For this review, take the finished solid that the model builds, in its own axes (mm). A direction names the side the tool comes from. Round coordinates to 2 decimals unless told otherwise and drop trailing zeros. Write each loop counter-clockwise with the first axis right and the second up, starting at its lowest first coordinate (ties: lowest second). Pieces come first, ordered by that corner, then holes. Notation, with made-up numbers: M 50,79.5 L 108,79.5 A20 ccw 108,84.5 Z; hole C 84.25,48.5 d11. An arc over 180 degrees is marked long. Use one line per item in the form item = value. Start each with the question number.
Item 1: Add section B-B (x = -8.25). State the section outline as (y, z) points.
Item 2: Add section D-D (x = 10.25). State the section outline as (y, z) points, and give its area (3 significant figures).
Item 3: For line 1 (Y direction, x = 7, z = 2.5); line 2 (Y direction, x = 9, z = 1.6); line 3 (Y direction, x = 2.75, z = 0.4), list the stretches that pass through material, from the lowest coordinate up. Write a range as [from, to].
Item 4: Add section A-A (z = 1.55). Count the separate pieces of the cut face and the enclosed holes in it, and give its area (3 significant figures).
Item 5: Add section C-C (y = 1.5). State the section outline as (x, z) points (3 decimals).
Item 6: Draft analysis for pull direction X (two halves, no side actions). For faces 4 (the flat face through (7, 0, 3.5)), 5 (the cylindrical face through (11.859, 22.797, 1.726)), 6 (the flat face through (-0.1, 1.2, 2)), state which applies: released by +X, released by -X, zero draft, split by the parting line, or undercut.
Item 7: For faces 1 (the flat face through (0, -24, 2)), 2 (the flat face through (-4.25, 0, 3)), 3 (the flat face through (0, -5, 1)), list the 3-axis set-ups (+Z, -Z, +X, -X, +Y, -Y) from which the entire face can be reached by the end or side of a thin tool; tool diameter is ignored.
from build123d import *

# Parameters (mm, degrees)
F0_R     = 1.75
F0_W     = 12
F0_H     = 10
F1_DEPTH = 2
F2_R     = 1.75
F3_DEPTH = 1.5
F4_R     = 1.125
F5_DEPTH = 60
F6_W     = 8.5
F6_H     = 2
F7_DEPTH = 5


with BuildPart() as f1:
    # F0 (on Top) → F1 (new body)
    with BuildSketch(Plane.XY):
        with BuildLine():
            ThreePointArc((-13, -20), (-11.828427, -22.828427), (-9, -24))
            Line((-9, -24), (9, -24))
            ThreePointArc((9, -24), (11.828427, -22.828427), (13, -20))
            Line((13, -20), (13, 20))
            ThreePointArc((13, 20), (11.828427, 22.828427), (9, 24))
            Line((9, 24), (-9, 24))
            ThreePointArc((-9, 24), (-11.828427, 22.828427), (-13, 20))
            Line((-13, 20), (-13, -20))
        make_face()
        with Locations((-9, -20)):
            Circle(F0_R, mode=Mode.SUBTRACT)
        with Locations((-7, -7)):
            Circle(F0_R, mode=Mode.SUBTRACT)
        with Locations((9, -20)):
            Circle(F0_R, mode=Mode.SUBTRACT)
        with Locations((7, -7)):
            Circle(F0_R, mode=Mode.SUBTRACT)
        with Locations((-7, 7)):
            Circle(F0_R, mode=Mode.SUBTRACT)
        with Locations((-9, 20)):
            Circle(F0_R, mode=Mode.SUBTRACT)
        Rectangle(F0_W, F0_H, mode=Mode.SUBTRACT)
        with Locations((7, 7)):
            Circle(F0_R, mode=Mode.SUBTRACT)
        with Locations((9, 20)):
            Circle(F0_R, mode=Mode.SUBTRACT)
    extrude(amount=F1_DEPTH)

    # F2 (on face) → F3 (join)
    with BuildSketch(Plane.XY.offset(2)):
        with BuildLine():
            ThreePointArc((-13, -20), (-11.828427, -22.828427), (-9, -24))
            Line((-9, -24), (9, -24))
            ThreePointArc((9, -24), (11.828427, -22.828427), (13, -20))
            Line((13, -20), (13, 20))
            ThreePointArc((13, 20), (11.828427, 22.828427), (9, 24))
            Line((9, 24), (-9, 24))
            ThreePointArc((-9, 24), (-11.828427, 22.828427), (-13, 20))
            Line((-13, 20), (-13, -20))
        make_face()
        with Locations((-9, -20)):
            Circle(F2_R, mode=Mode.SUBTRACT)
        with Locations((-7, -7)):
            Circle(F2_R, mode=Mode.SUBTRACT)
        with Locations((9, -20)):
            Circle(F2_R, mode=Mode.SUBTRACT)
        with Locations((7, -7)):
            Circle(F2_R, mode=Mode.SUBTRACT)
        with Locations((-7, 7)):
            Circle(F2_R, mode=Mode.SUBTRACT)
        with Locations((-9, 20)):
            Circle(F2_R, mode=Mode.SUBTRACT)
        with Locations((7, 7)):
            Circle(F2_R, mode=Mode.SUBTRACT)
        with Locations((9, 20)):
            Circle(F2_R, mode=Mode.SUBTRACT)
    extrude(amount=F3_DEPTH)


with BuildPart() as f5:
    # F4 (on face) → F5 (new body)
    with BuildSketch(Plane.XZ.offset(24)):
        with Locations((0, 3.5)):
            Circle(F4_R)
    extrude(amount=-F5_DEPTH)


with BuildPart() as f7:
    # F6 (on face) → F7 (new body)
    with BuildSketch(Plane.XY.offset(3.5)):
        Rectangle(F6_W, F6_H)
    extrude(amount=-F7_DEPTH)


with BuildPart() as f1_1:
    add(f1.part)

    # F8: cut F5, F7
    add(f5.part, mode=Mode.SUBTRACT)
    add(f7.part, mode=Mode.SUBTRACT)


solid = f1_1.part
Calculated:
q1.outline = M -24,0 L -21.58,0 L -21.58,3.5 L -24,3.5 Z; M -18.42,0 L -8.22,0 L -8.22,3.5 L -18.42,3.5 Z; M -5.78,0 L 5.78,0 L 5.78,3.5 L -5.78,3.5 Z; M 8.22,0 L 18.42,0 L 18.42,3.5 L 8.22,3.5 Z; M 21.58,0 L 24,0 L 24,3.5 L 21.58,3.5 Z
q2.outline = M -23.8,0 L -21.22,0 L -21.22,3.5 L -23.8,3.5 Z; M -18.78,0 L 18.78,0 L 18.78,3.5 L -18.78,3.5 Z; M 21.22,0 L 23.8,0 L 23.8,3.5 L 21.22,3.5 Z
q2.area = 149 mm^2
q3.line_1 = [-24, -8.75], [-5.25, 5.25], [8.75, 24]
q3.line_2 = [-24, -21.75], [-18.25, 18.25], [21.75, 24]
q3.line_3 = [-24, -5], [5, 24]
q4.separate_pieces = 1
q4.enclosed_holes = 9
q4.area = 1,040 mm^2
q5.outline = M -13,0 L -6,0 L -6,2 L 6,2 L 6,0 L 13,0 L 13,3.5 L 1.125,3.5 A1.125 cw -1.125,3.5 L -13,3.5 Z
q6.face_4 = zero draft
q6.face_5 = released by +X
q6.face_6 = undercut
q7.face_1 = +Z, -Z, +X, -X, -Y
q7.face_2 = +Z, -Z
q7.face_3 = -Z
